Design review of the part built by this model. Coordinates are the model's own, in mm. A direction names the side the tool comes from. Give positions to 0.01 mm unless a question says otherwise; leave off trailing zeros. Write each loop counter-clockwise with the first axis right and the second up, starting at its lowest first coordinate (ties: lowest second). Pieces come first, ordered by that corner, then holes. Notation, with made-up numbers: M -28,-22 L 25,-22 A19 ccw 25,-7 Z; hole C 20,-35.5 d11. An arc over 180 degrees is marked long. Use a Markdown table: item, result. Add a question column.
```python
from build123d import *

# Parameters (mm, degrees)
SKETCH_R     = 42.5
PAD_DEPTH    = 90
FILLET_R     = 5
FILLET001_R  = 5
SKETCH001_R  = 16.5
PAD001_DEPTH = 8
FILLET002_R  = 3
SKETCH002_R  = 4
PAD002_DEPTH = 32
PAD003_DEPTH = 6
SKETCH004_R  = 16.5
PAD004_DEPTH = 10
FILLET003_R  = 3
SKETCH005_R  = 2.5
PAD005_DEPTH = 11


with BuildPart() as part:
    # Sketch → Pad (new body)
    with BuildSketch(Plane.XZ):
        Circle(SKETCH_R)
    extrude(amount=PAD_DEPTH)

    # Fillet
    fillet_edges = [part.edges().sort_by_distance(p)[0] for p in [
        (-42.5, -90, 0),
    ]]
    fillet(fillet_edges, radius=FILLET_R)

    # Fillet001
    fillet001_edges = [part.edges().sort_by_distance(p)[0] for p in [
        (-42.5, 0, 0),
    ]]
    fillet(fillet001_edges, radius=FILLET001_R)

    # Sketch001 (on Face5 of Fillet001) → Pad001 (join)
    with BuildSketch(Plane.XZ.offset(90)):
        Circle(SKETCH001_R)
    extrude(amount=PAD001_DEPTH)

    # Fillet002
    fillet002_edges = [part.edges().sort_by_distance(p)[0] for p in [
        (-16.5, -98, 0),
    ]]
    fillet(fillet002_edges, radius=FILLET002_R)

    # Sketch002 (on Face4 of Fillet002) → Pad002 (join)
    with BuildSketch(Plane.XZ.offset(98)):
        Circle(SKETCH002_R)
    extrude(amount=PAD002_DEPTH)

    # Sketch003 (on Face10 of Pad002) → Pad003 (join)
    with BuildSketch(Plane(origin=(0, 0, 0), x_dir=(1, 0, 0), z_dir=(0, 1, 0))):
        with BuildLine():
            Line((-20.922476, 21.5), (20.922476, 21.5))
            ThreePointArc((20.922476, -21.5), (30, 0), (20.922476, 21.5))
            Line((-20.922476, -21.5), (20.922476, -21.5))
            ThreePointArc((-20.922476, 21.5), (-30, 0), (-20.922476, -21.5))
        make_face()
    extrude(amount=PAD003_DEPTH)

    # Sketch004 (on Face15 of Pad003) → Pad004 (join)
    with BuildSketch(Plane(origin=(0, 6, 0), x_dir=(1, 0, 0), z_dir=(0, 1, 0))):
        Circle(SKETCH004_R)
    extrude(amount=PAD004_DEPTH)

    # Fillet003
    fillet003_edges = [part.edges().sort_by_distance(p)[0] for p in [
        (-16.5, 16, 0),
    ]]
    fillet(fillet003_edges, radius=FILLET003_R)

    # Sketch005 (on Face13 of Fillet003) → Pad005 (join)
    with BuildSketch(Plane.XZ.offset(90)):
        with Locations((-35, 0)):
            Circle(SKETCH005_R)
        with Locations((35, 0)):
            Circle(SKETCH005_R)
    extrude(amount=PAD005_DEPTH)


solid = part.part
```
(1) Add section A-A on x = 0. Give the boundary of the cut face in (y, z).
(2) Add section B-B on y = -12.5. Give the boundary of the cut face in (x, z).
(3) Wall thickness on L1, parallel to Y at x = -4, z = -31; L2, parallel to Z at x = 1, y = -64.5; L3, parallel to Y at x = 28, z = 1: over which ranges is each line inside the solid? List them lowest first.
(4) Machinability: for faces 1 (the cylindrical face through (-0.867, -113.776, -3.905)), 2 (the flat face through (0, 3, -21.5)), 3 (the cylindrical face through (-30, 3, 0)), 4 (the flat face through (35, -101, 0)), 5 (the flat face through (-1, 0, -24)), which of the approach directions +Z, -Z, +X, -X, +Y, -Y give a long, thin tool a straight path to every point of the face, cutting with its end or side? Answer none if there is none.
(5) For pin 1 (5 mm diameter, centred on x = 0, y = 4, fed in from +Z); pin 2 (5.5 mm diameter, centred on x = -35.5, z = 0, fed in from -Y); pin 3 (2 mm diameter, centred on x = -22.5, y = -50, fed in from -Z), all flat-tipped, find the tip position at first contact; note any pin that passes through.
(6) The part is to be moulded in two halves that separate along X. For faces 6 (the cylindrical face through (30, 3, 0)), 7 (the cylindrical face through (-32.69, -95.42, -0.96)), 8 (the cylindrical face through (37.31, -95.42, -0.96)), 9 (the flat face through (0, 3, 21.5)), say which applies: released by +X, released by -X, zero draft, split by the parting line, or undercut.
From the geometry:
| question | item | result |
|---|---|---|
| 1 | outline | M -130,-4 L -98,-4 L -98,-13.5 A3 ccw -95,-16.5 L -90,-16.5 L -90,-37.5 A5 ccw -85,-42.5 L -5,-42.5 A5 ccw 0,-37.5 L 0,-21.5 L 6,-21.5 L 6,-16.5 L 13,-16.5 A3 ccw 16,-13.5 L 16,13.5 A3 ccw 13,16.5 L 6,16.5 L 6,21.5 L 0,21.5 L 0,37.5 A5 ccw -5,42.5 L -85,42.5 A5 ccw -90,37.5 L -90,16.5 L -95,16.5 A3 ccw -98,13.5 L -98,4 L -130,4 Z |
| 2 | outline | C 0,0 d85 |
| 3 | L1 | y = -90 to 0 |
| 3 | L2 | z = -42.49 to 42.49 |
| 3 | L3 | y = -90 to 6 |
| 4 | face 1 | -Y |
| 4 | face 2 | -Z, +X, -X, +Y |
| 4 | face 3 | -X, +Y |
| 4 | face 4 | +Z, -Z, +X, -Y |
| 4 | face 5 | +Y |
| 5 | pin 1 | stops at z = 21.5 |
| 5 | pin 2 | stops at y = -101 |
| 5 | pin 3 | stops at z = -36.66 |
| 6 | face 6 | released by +X |
| 6 | face 7 | undercut |
| 6 | face 8 | undercut |
| 6 | face 9 | zero draft |
